Read the model definition and answer for the solid it produces. Units are mm, in the model's axes. A direction names the side the tool comes from. Coordinates: 2 decimals unless noted, no trailing zeros. Loops run counter-clockwise (first coordinate to the right, second up) from the corner with the lowest first, then second, coordinate; pieces in that order, holes last. Notation, with made-up numbers: M -4,-29 L 20,-29 A30 ccw 20,1 Z; hole C -31,35 d2. An arc over 180 degrees is marked long. One line per item, written item: value. Start each with the question number.
1. The part is cut by section A-A (y = -1.5). Write down the section's boundary in (x, z).
2. Consider probe 1 along Z at (x, y) = (0.4, -1.5); probe 2 along Z at (x, y) = (-1.5, -1.25); probe 3 along X at (y, z) = (-4.5, 5). Determine where each line is inside the solid, lowest interval first.
3. Flat-ended cylindrical pins translate along their axes: pin 1 (2 mm diameter, centred on x = 0.5, y = 0, fed in from +Z) (3 decimals); pin 2 (1 mm diameter, centred on x = -1.5, z = -1, fed in from -Y). Find the tip coordinate at first contact, or state that the pin passes through.
4. The part is cut by section B-B (x = 0.3). Write down the section's boundary in (y, z), then the cut area to 3 significant figures.
5. Determine the mould class of faces 1 (the face through (0, -5.25, -5)), 2 (the face through (-1, 0, 3.75)) for opening direction Z: +Z half, -Z half, draft (parallel to the pull), parting line (faces both ways), or undercut.
6. For faces 3 (the face through (-1, 0, -3.75)), 4 (the face through (0, -5.25, 5)), determine the directions among +Z, -Z, +X, -X, +Y, -Y from which every point of the face is accessible in a straight line to the end or side of a thin tool.
7. The part is cut by section D-D (x = -0.85). Write down the section's boundary in (y, z).
8. The part is cut by section C-C (z = -0.5). Write down the section's boundary in (x, y), then the cut area to 3 significant figures.
```python
from build123d import *

# Parameters (mm, degrees)
SKETCH_1_R        = 2.25
EXTRUDE_1_DEPTH   = 3.75
SKETCH_4_R        = 0.6
EXTRUDE_2_DEPTH   = 3
EXTRUDE_2_2_DEPTH = 3
SKETCH_2_R        = 0.6
SKETCH_7_R        = 0.6


with BuildPart() as part:
    # Sketch 1 → Extrude 1 (new, symmetric)
    with BuildSketch(Plane.XY):
        Circle(SKETCH_1_R)
    extrude(amount=EXTRUDE_1_DEPTH, both=True)



with BuildPart() as body_2:
    # Sketch 4 → Extrude 2 (new body)
    with BuildSketch(Plane(origin=(0, -2.25, 0), x_dir=(-1, 0, 0), z_dir=(0, -1, 0))):
        with Locations(Location((0, -5, 0), (0, 0, 90))):
            Circle(SKETCH_4_R)
    extrude(amount=EXTRUDE_2_DEPTH)


with BuildPart() as body_3:
    # Sketch 4 → Extrude 2 2 (new body)
    with BuildSketch(Plane(origin=(0, -2.25, 0), x_dir=(-1, 0, 0), z_dir=(0, -1, 0))):
        with Locations(Location((0, 5, 0), (0, 0, 90))):
            Circle(SKETCH_4_R)
    extrude(amount=EXTRUDE_2_2_DEPTH)


with BuildPart() as part_1:
    add(part.part)

    add(body_2.part)  # Sweep 2 merges body 2
    # Sweep 2: sweep along a path in Sketch 5
    with BuildLine(Plane(origin=(0, 0, 0), x_dir=(0, 0, -1), z_dir=(1, 0, 0))) as sweep_2_path:
        Line((-3.75, 0), (-4, 0))
        ThreePointArc((-4, 0), (-4.707106781, -0.292893219), (-5, -1))
        Line((-5, -1), (-5, -3.422153909))
    # Sketch 2 → Sweep 2 (sweep)
    with BuildSketch(Plane.XY.offset(3.75)):
        Circle(SKETCH_2_R)
    sweep(path=sweep_2_path.line)


    add(body_3.part)  # Sweep 3 merges body 3
    # Sweep 3: sweep along a path in Sketch 6
    with BuildLine(Plane(origin=(0, 0, 0), x_dir=(0, 0, -1), z_dir=(1, 0, 0))) as sweep_3_path:
        Line((3.75, 0), (4, 0))
        ThreePointArc((4, 0), (4.707106781, -0.292893219), (5, -1))
        Line((5, -1), (5, -3.141146962))
    # Sketch 7 → Sweep 3 (sweep)
    with BuildSketch(Plane(origin=(0, 0, -3.75), x_dir=(-1, 0, 0), z_dir=(0, 0, -1))):
        Circle(SKETCH_7_R)
    sweep(path=sweep_3_path.line)


solid = part_1.part
```
Answer block:
1. outline: M -1.68,-3.75 L 1.68,-3.75 L 1.68,3.75 L -1.68,3.75 Z; C 0,-5 d1.2; C 0,5 d1.2
2. probe 1: z = -5.45 to -4.55, -3.75 to 3.75, 4.55 to 5.45
2. probe 2: z = -3.75 to 3.75
2. probe 3: x = -0.6 to 0.6
3. pin 1: stops at z = 5.595
3. pin 2: stops at y = -2.02
4. outline: M -5.25,-5.52 L -1,-5.52 A1.52 ccw 0.52,-4 L 0.52,-3.75 L 2.23,-3.75 L 2.23,3.75 L 0.52,3.75 L 0.52,4 A1.52 ccw -1,5.52 L -5.25,5.52 L -5.25,4.48 L -1,4.48 A0.48 cw -0.52,4 L -0.52,3.75 L -2.23,3.75 L -2.23,-3.75 L -0.52,-3.75 L -0.52,-4 A0.48 cw -1,-4.48 L -5.25,-4.48 Z
4. area: 46.1 mm2
5. face 1: draft
5. face 2: undercut
6. face 3: none
6. face 4: +Z, -Z, +X, -X, -Y
7. outline: M -2.08,-3.75 L 2.08,-3.75 L 2.08,3.75 L -2.08,3.75 Z
8. outline: C 0,0 d4.5
8. area: 15.9 mm2
